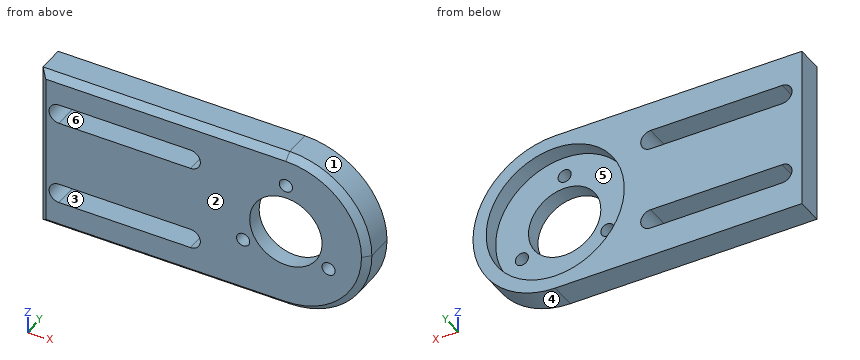
```python
from build123d import *

# Parameters (mm, degrees)
SKETCH1_W               = 100
SKETCH1_H               = 50
BOSS_EXTRUDE1_DEPTH     = 10
FILLET1_R               = 25
CUT_EXTRUDE1_DEPTH      = 113.249721603
CUT_EXTRUDE1_DEPTH_BACK = 113.249721603
SKETCH2_R               = 11
SKETCH2_R_2             = 2
SKETCH3_R               = 21
CUT_EXTRUDE2_DEPTH      = 5
CUT_EXTRUDE3_DEPTH      = 113.249721603
CUT_EXTRUDE3_DEPTH_BACK = 113.249721603
CHAMFER1_SIZE           = 2


with BuildPart() as part:
    # Sketch1 → Boss-Extrude1 (new body)
    with BuildSketch(Plane(origin=(0, 0, 0), x_dir=(1, 0, 0), z_dir=(0, 1, 0))):
        with Locations((50, 25)):
            Rectangle(SKETCH1_W, SKETCH1_H)
    extrude(amount=BOSS_EXTRUDE1_DEPTH)

    # Fillet1
    fillet1_edges = [part.edges().sort_by_distance(p)[0] for p in [
        (100, 5, -50),
        (100, 5, 0),
    ]]
    fillet(fillet1_edges, radius=FILLET1_R - 0.0001)  # a hair under: the kernel refuses the full size

    # Sketch2 → Cut-Extrude1 (cut, two sides: drawn at the far end of the back side and taken through both)
    with BuildSketch(Plane(origin=(0, 0, 0), x_dir=(1, 0, 0), z_dir=(0, 1, 0)).offset(-CUT_EXTRUDE1_DEPTH_BACK)):
        with Locations(Location((75, 25, 0), (0, 0, 90))):
            Circle(SKETCH2_R)
        with Locations(Location((75, 10, 0), (0, 0, 90))):
            Circle(SKETCH2_R_2)
        with Locations(Location((62.009618943, 32.5, 0), (0, 0, 90))):
            Circle(SKETCH2_R_2)
        with Locations(Location((87.990381057, 32.5, 0), (0, 0, 90))):
            Circle(SKETCH2_R_2)
    extrude(amount=CUT_EXTRUDE1_DEPTH + CUT_EXTRUDE1_DEPTH_BACK, mode=Mode.SUBTRACT)

    # Sketch3 → Cut-Extrude2 (cut)
    with BuildSketch(Plane(origin=(0, 10, 0), x_dir=(1, 0, 0), z_dir=(0, 1, 0))):
        with Locations(Location((75, 25, 0), (0, 0, 270))):
            Circle(SKETCH3_R)
    extrude(amount=-CUT_EXTRUDE2_DEPTH, mode=Mode.SUBTRACT)

    # Sketch4 → Cut-Extrude3 (cut, two sides: drawn at the far end of the back side and taken through both)
    with BuildSketch(Plane(origin=(0, 0, 0), x_dir=(1, 0, 0), z_dir=(0, 1, 0)).offset(-CUT_EXTRUDE3_DEPTH_BACK)):
        with BuildLine():
            Line((6, 15), (46, 15))
            ThreePointArc((46, 15), (49, 12), (46, 9))
            Line((46, 9), (6, 9))
            ThreePointArc((6, 9), (3, 12), (6, 15))
        make_face()
        with BuildLine():
            Line((46, 35), (6, 35))
            ThreePointArc((6, 35), (3, 38), (6, 41))
            Line((6, 41), (46, 41))
            ThreePointArc((46, 41), (49, 38), (46, 35))
        make_face()
    extrude(amount=CUT_EXTRUDE3_DEPTH + CUT_EXTRUDE3_DEPTH_BACK, mode=Mode.SUBTRACT)

    # Chamfer1
    chamfer1_edges = [part.edges().sort_by_distance(p)[0] for p in [
        (37.50005, 0, -50),
        (92.677698819, 0, -7.322301181),
        (92.677698819, 0, -42.677698819),
        (37.50005, 0, 0),
        (0, 0, -25),
    ]]
    chamfer(chamfer1_edges, length=CHAMFER1_SIZE)


solid = part.part
```
Design review of the part built by this model. Coordinates are the model's own, in mm. Face numbers are marked on the shaded views. A direction names the side the tool comes from. Give positions to 0.01 mm unless a question says otherwise; leave off trailing zeros. Loops run counter-clockwise (first coordinate to the right, second up) from the corner with the lowest first, then second, coordinate; pieces in that order, holes last. Notation, with made-up numbers: (51, 78.5) -> (100, 78.5) arc R19 cw to (100, 85.5) -> close; hole circle Ø5 at (26, -6.5). An arc over 180 degrees is marked (long way). Write each question's results on one line, items separated by ' | '.
Q1. Take a section at A-A, the plane x = 7.5. Write out the cut boundary in (y, z), plus the area to 3 significant figures.
Reply:
outline: (0, -48) -> (2, -50) -> (10, -50) -> (10, -41) -> (0, -41) -> close; (0, -35) -> (10, -35) -> (10, -15) -> (0, -15) -> close; (0, -9) -> (10, -9) -> (10, 0) -> (2, 0) -> (0, -2) -> close | area: 376 mm²
Q2. For pin 1 Ø3 at (x, z) = (62.01, -32.5) entering from -Y; pin 2 Ø5 at (x, z) = (75, -10) entering from -Y, all flat-tipped, find the tip position at first contact; note any pin that passes through.
Reply:
pin 1: passes through | pin 2: stops at y = 0
Q3. The part is to be moulded in two halves that separate along X. For the marked faces 1, 2 and 3, say which applies: +X half, -X half, draft (parallel to the pull), parting line (faces both ways), or undercut.
Reply:
face 1: +X half | face 2: draft | face 3: undercut
Q4. Take a section at D-D, the plane x = 55.5. Write out the cut boundary in (y, z), plus the area to 3 significant figures.
Reply:
outline: (0, -48) -> (2, -50) -> (10, -50) -> (10, -32.79) -> (5, -32.79) -> (5, -17.21) -> (10, -17.21) -> (10, 0) -> (2, 0) -> (0, -2) -> close | area: 418 mm²
Q5. Machinability: for the marked faces 4, 5 and 6, which of the approach directions +Z, -Z, +X, -X, +Y, -Y give a long, thin tool a straight path to every point of the face, cutting with its end or side? Answer none if there is none.
Reply:
face 4: -Z, +X, +Y, -Y | face 5: +Y | face 6: +Y, -Y
Q6. Wall thickness on L1, parallel to Z at x = 26, y = 4; L2, parallel to X at y = 1.8, z = -10; L3, parallel to X at y = 5.25, z = -37: over which ranges is each line inside the solid? List them lowest first.
Reply:
L1: z = -50 to -41, -35 to -15, -9 to 0 | L2: x = 0.2 to 3.76, 48.24 to 73, 77 to 94.75 | L3: x = 0 to 3.17, 48.83 to 57.77, 92.23 to 96.93
Q7. Take a section at B-B, the plane y = 3. Give the number of separate pieces and of enclosed holes in the cut face, plus the area to 3 significant figures.
Reply:
separate pieces: 1 | enclosed holes: 6 | area: 3,780 mm²
